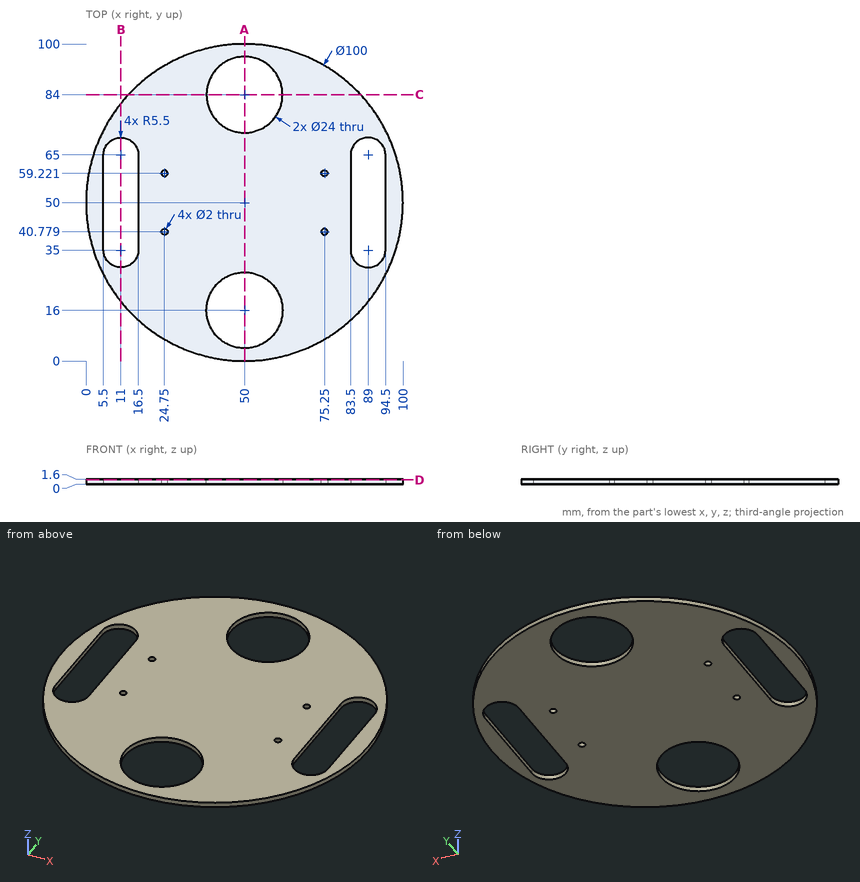
Geometry check sheet. Reference: drawing and pictorial views, mm from the part's lowest x, y, z. Round coordinates to 2 decimals unless told otherwise and drop trailing zeros. Write each loop counter-clockwise with the first axis right and the second up, starting at its lowest first coordinate (ties: lowest second). Pieces come first, ordered by that corner, then holes.
1. Section check A-A on x = 50. Enter the section's corners in (y, z), plus the area to 3 significant figures.
2. Section check D-D on z = 1.35. State how many separate pieces and enclosed holes the cut face has, plus the area to 3 significant figures.
3. Gauge pin test, flat ends, axial feed: P1, Ø0.8, axis at y = 45.5, z = 0.5, coming from the -X side; P2, Ø0.5, axis at y = 52.5, z = 1, coming from the +X side; P3, Ø0.8, axis at y = 52.5, z = 0.5, coming from the +X side. Record the tip position at first contact, or that the pin passes through.
4. Section check B-B on x = 11. Enter the section's corners in (y, z).
5. Section check C-C on y = 84. Enter the section's corners in (x, z).
6. Scan lines: L1, parallel to X at y = 51, z = 1.2; L2, parallel to Y at x = 75.25, z = 1; L3, parallel to Y at x = 75.5, z = 1.3. Record each from-to range of solid material in increasing order.
Answer:
1. outline: (0, 0) - (4, 0) - (4, 1.6) - (0, 1.6) - close; (28, 0) - (72, 0) - (72, 1.6) - (28, 1.6) - close; (96, 0) - (100, 0) - (100, 1.6) - (96, 1.6) - close
1. area: 83.2 mm2
2. separate pieces: 1
2. enclosed holes: 8
2. area: 6,090 mm2
3. P1: stops at x = 0.17
3. P2: stops at x = 99.95
3. P3: stops at x = 99.96
4. outline: (18.71, 0) - (29.5, 0) - (29.5, 1.6) - (18.71, 1.6) - close; (70.5, 0) - (81.29, 0) - (81.29, 1.6) - (70.5, 1.6) - close
5. outline: (13.34, 0) - (38, 0) - (38, 1.6) - (13.34, 1.6) - close; (62, 0) - (86.66, 0) - (86.66, 1.6) - (62, 1.6) - close
6. L1: x = 0.01 to 5.5, 16.5 to 83.5, 94.5 to 99.99
6. L2: y = 6.84 to 39.78, 41.78 to 58.22, 60.22 to 93.16
6. L3: y = 6.99 to 39.81, 41.75 to 58.25, 60.19 to 93.01
